Check sheet for the modelled part. Datum: model origin and axes. Units: mm. Coordinates: 2 decimals unless noted, no trailing zeros. Loops run counter-clockwise (first coordinate to the right, second up) from the corner with the lowest first, then second, coordinate; pieces in that order, holes last. Notation, with made-up numbers: (82, 55.5) - (88, 55.5) arc R13 cw to (88, 65.5) - close; hole circle Ø2 at (-35, -23). An arc over 180 degrees is marked (long way). Write each question's results on one line, items separated by ' | '. Start each with the question number.
1. Cross-section at D-D (x = 560). Record the cut outline in (y, z).
2. Cross-section at B-B (x = 475). Record the cut outline in (y, z).
3. Cross-section at A-A (z = -13.1). Record the cut outline in (x, y).
4. Draft check along X on faces 1 (the face through (0, 13, -38)), 2 (the face through (130, 12.9, -14.7)), 3 (the face through (566.438, 12.878, -65.128)), 4 (the face through (296, 13, -76.2)). Enter one of: released by +X, released by -X, zero draft, split by the parting line, or undercut.
5. Cross-section at C-C (y = 8.5). Give the number of separate pieces and of enclosed holes in the cut face, and give its area (3 significant figures).
6. Thickness scan on line 1 (X direction, y = 18.5, z = -13.1); line 2 (Z direction, x = 475, y = 13.75); line 3 (Z direction, x = 560, y = 18.5). Record the ranges inside material, lowest first. Write a range as [from, to].
```python
from build123d import *

# Parameters (mm, degrees)
SKETCH1_W           = 600
SKETCH1_H           = 76.2
BOSS_EXTRUDE1_DEPTH = 25.4
SKETCH2_R           = 6.75
CUT_EXTRUDE1_DEPTH  = 25.4
SKETCH3_R           = 5.25
CUT_EXTRUDE2_DEPTH  = 25.4


with BuildPart() as part:
    # Sketch1 → Boss-Extrude1 (new body)
    with BuildSketch(Plane(origin=(0, 0, 0), x_dir=(1, 0, 0), z_dir=(0, 1, 0))):
        with Locations((300, 38.1)):
            Rectangle(SKETCH1_W, SKETCH1_H)
    extrude(amount=BOSS_EXTRUDE1_DEPTH)

    # Sketch2 → Cut-Extrude1 (cut)
    with BuildSketch(Plane(origin=(0, 25.4, 0), x_dir=(1, 0, 0), z_dir=(0, 1, 0))):
        with Locations((40, 63.1)):
            Circle(SKETCH2_R)
        with Locations((40, 13.1)):
            Circle(SKETCH2_R)
        with Locations((560, 13.1)):
            Circle(SKETCH2_R)
        with Locations((560, 63.1)):
            Circle(SKETCH2_R)
    extrude(amount=-CUT_EXTRUDE1_DEPTH, mode=Mode.SUBTRACT)

    # Sketch3 → Cut-Extrude2 (cut)
    with BuildSketch(Plane(origin=(0, 25.4, 0), x_dir=(1, 0, 0), z_dir=(0, 1, 0))):
        with Locations((125, 63.1)):
            Circle(SKETCH3_R)
        with Locations((125, 13.1)):
            Circle(SKETCH3_R)
        with Locations((475, 13.1)):
            Circle(SKETCH3_R)
        with Locations((475, 63.1)):
            Circle(SKETCH3_R)
    extrude(amount=-CUT_EXTRUDE2_DEPTH, mode=Mode.SUBTRACT)


solid = part.part
```
Established:
1) outline: (0, -76.2) - (25.4, -76.2) - (25.4, -69.85) - (0, -69.85) - close; (0, -56.35) - (25.4, -56.35) - (25.4, -19.85) - (0, -19.85) - close; (0, -6.35) - (25.4, -6.35) - (25.4, 0) - (0, 0) - close
2) outline: (0, -76.2) - (25.4, -76.2) - (25.4, -68.35) - (0, -68.35) - close; (0, -57.85) - (25.4, -57.85) - (25.4, -18.35) - (0, -18.35) - close; (0, -7.85) - (25.4, -7.85) - (25.4, 0) - (0, 0) - close
3) outline: (0, 0) - (33.25, 0) - (33.25, 25.4) - (0, 25.4) - close; (46.75, 0) - (119.75, 0) - (119.75, 25.4) - (46.75, 25.4) - close; (130.25, 0) - (469.75, 0) - (469.75, 25.4) - (130.25, 25.4) - close; (480.25, 0) - (553.25, 0) - (553.25, 25.4) - (480.25, 25.4) - close; (566.75, 0) - (600, 0) - (600, 25.4) - (566.75, 25.4) - close
4) face 1: released by -X | face 2: undercut | face 3: undercut | face 4: zero draft
5) separate pieces: 1 | enclosed holes: 8 | area: 44,800 mm^2
6) line 1: [0, 33.25], [46.75, 119.75], [130.25, 469.75], [480.25, 553.25], [566.75, 600] | line 2: [-76.2, -68.35], [-57.85, -18.35], [-7.85, 0] | line 3: [-76.2, -69.85], [-56.35, -19.85], [-6.35, 0]
